Source: CAD feature listing. Evaluate the final solid. Frame: model axes, mm. A direction names the side the tool comes from. Give positions to 0.01 mm unless a question says otherwise; leave off trailing zeros. Loops run counter-clockwise (first coordinate to the right, second up) from the corner with the lowest first, then second, coordinate; pieces in that order, holes last. Notation, with made-up numbers: M 51,-16.75 L 77,-16.75 A9 ccw 77,-4.75 Z; hole C 44,42 d6. An arc over 180 degrees is marked long. Answer in a Markdown table with one row per item.
Autodesk Inventor part; units mm, degrees
ref_plane "YZ Plane" through (0, 0, 0) normal (1, 0, 0) x (0, 1, 0)
ref_plane "XZ Plane" through (0, 0, 0) normal (0, 1, 0) x (-1, 0, 0)
ref_plane "XY Plane" through (0, 0, 0) normal (0, 0, 1) x (1, 0, 0)
sketch "草圖1" plane through (0, 0, 0) normal (0, 1, 0) x (-1, 0, 0)
  line L0 (0, 0) -> (42, 0)
  line L1 (42, 0) -> (42, 12)
  line L2 (42, 12) -> (0, 12)
  line L3 (0, 12) -> (0, 0)
  line L4 (0, 0) -> (-8.5, 0)
  line L5 (-10, 1.5) -> (-10, 1.5)
  line L6 (-8.5, 3) -> (0, 3)
  line L7 (0, 3) -> (0, 0)
  line L8 (30, 0) -> (42, 0)
  line L9 (42, 0) -> (42, -6)
  line L10 (36, -12) -> (36, -12)
  line L11 (30, -6) -> (30, 0)
  arc A0 (30, -6) -> (36, -12) centre (36, -6) ccw
  arc A1 (36, -12) -> (42, -6) centre (36, -6) ccw
  arc A2 (-8.5, 3) -> (-10, 1.5) centre (-8.5, 1.5) ccw
  arc A3 (-10, 1.5) -> (-8.5, 0) centre (-8.5, 1.5) ccw
  point P0 (-10, 3)
  point P1 (-10, 0)
  point P2 (42, -12)
  point P3 (30, -12)
  dimension "d0" = 42
  dimension "d2" = 10
  dimension "d3" = 3
  dimension "d4" = 12
  dimension "d6" = 12
  dimension "d7" = 12
  dimension "d8" = 6
  dimension "d9" = 1.5
extrude "擠出1" add sketch "草圖1" along normal blind 12
fillet "圓角1" radius 3 4 edges at (-42, 6, 12) (-30, 6, 0) (0, 6, 3) (0, 6, 12)
sketch "草圖2" plane through (0, 12, 0) normal (0, 1, 0) x (1, 0, 0)
  line L0 (-42, 6) -> (-42, -9)
  line L1 (-39, -12) -> (-3, -12)
  point P0 (0, 0)
  point P1 (-36, -6)
  dimension "d13" = 6
  dimension "d14" = 6
hole "孔1" at (-36, 12, 6) direction (0, -1, 0) diameter 3 end through all counterbore diameter 7 counterbore depth 2
sketch "草圖3" plane through (8.5, 0, 0) normal (0, 0, -1) x (-1, 0, 0)
  line L0 (35.5, 12) -> (35.5, 0)
  line L1 (0, 0) -> (35.5, 0)
  line L2 (35.5, 9) -> (50.5, 9)
  line L3 (50.5, 9) -> (50.5, 3)
  line L4 (50.5, 3) -> (35.5, 3)
  line L5 (35.5, 3) -> (35.5, 9)
  point P0 (8.5, 0)
  dimension "d22" = 6
  dimension "d24" = 15
  dimension "d25" = 3
extrude "擠出2" cut sketch "草圖3" along normal blind 12
sketch "草圖4" plane through (0, 12, 0) normal (0, 1, 0) x (1, 0, 0)
  line L0 (-30, 3) -> (-30, 6)
  point P0 (0, 0)
  point P1 (-34, 6)
  dimension "d28" = 4
hole "孔2" at (-34, 12, -6) direction (0, -1, 0) diameter 3.242 end through all counterbore diameter 7.5 counterbore depth 2
sketch "草圖5" plane through (-39, 0, 12) normal (0, 0, 1) x (1, 0, 0)
  line L0 (-3, 12) -> (-3, 0)
  point P0 (39, 0)
  point P1 (12, 6)
  dimension "d36" = 15
hole "孔3" at (-27, 6, 12) direction (0, 0, -1) diameter 2.5 end through all
chamfer "倒角1" distance 0.25 angle 45 2 edges at (-27, 7.25, 12) (-27, 7.25, 0)
sketch "草圖6" plane through (-39, 0, 12) normal (0, 0, 1) x (1, 0, 0)
  line L0 (-3, 12) -> (-3, 0)
  point P0 (39, 0)
  point P1 (29, 6)
  dimension "d47" = 32
hole "孔4" at (-10, 6, 12) direction (0, 0, -1) diameter 3.242 end through all
properties part number "extruder_lever"
1) Material intervals for L1, parallel to Z at x = -36, y = 8.5; L2, parallel to Y at x = -27, z = 5.5; L3, parallel to Z at x = -23, y = 2.5, sorted ascending.
Reply:
| item | result |
|---|---|
| L1 | z = 0 to 4.5, 7.5 to 12 |
| L2 | y = 0 to 4.75, 7.25 to 12 |
| L3 | z = 0 to 12 |
2) Section D-D, the plane z = 3.75. Return loops of the section in (x, y).
Reply:
| item | result |
|---|---|
| outline | M -42,0 L 1.02,0 L 1.02,12 L -33.32,12 L -33.32,10 L -38.68,10 L -38.68,12 L -42,12 Z; hole C -27,6 d2.5; hole C -10,6 d3.24 |
3) Section A-A, the plane y = 6. Return loops of the section in (x, z).
Reply:
| item | result |
|---|---|
| outline | M -42,0 L -28.5,0 L -28.25,0.25 L -28.25,11.75 L -28.5,12 L -39,12 A3 ccw -42,9 Z; M -25.75,0.25 L -25.5,0 L -11.62,0 L -11.62,12 L -25.5,12 L -25.75,11.75 Z; M -8.38,0 L 8.5,0 A1.5 ccw 8.5,3 L 3,3 A3 cw 0,6 L 0,9 A3 ccw -3,12 L -8.38,12 Z; hole C -36,6 d3 |
4) Set-up query: faces 1 (the flat face through (-16, 6, 0)), 2 (the cylindrical face through (-39.47, 10.99, 5.54)), 3 (the flat face through (-30, 10, -5)), 4 (the flat face through (6, 6, 3)). Return all of +Z, -Z, +X, -X, +Y, -Y with unobstructed straight access to the full face (end or side cutting, diameter ignored); none if empty.
Reply:
| item | result |
|---|---|
| face 1 | -Z, +X |
| face 2 | +Y |
| face 3 | -Z, +X, +Y, -Y |
| face 4 | +Z, +X, +Y, -Y |
5) Section B-B, the plane x = -10. Return loops of the section in (y, z).
Reply:
| item | result |
|---|---|
| outline | M 0,0 L 4.38,0 L 4.38,12 L 0,12 Z; M 7.62,0 L 12,0 L 12,12 L 7.62,12 Z |
6) Pin query (flat end, axial travel): pin 1 Ø3.5 at (y, z) = (2, -4.5) entering from +X; pin 2 Ø1.5 at (y, z) = (4, 7.5) entering from +X; pin 3 Ø5 at (x, z) = (-34, -6) entering from +Y; pin 4 Ø1.8 at (x, z) = (-36, 6) entering from -Y. Return the tip coordinate at first contact, or that it passes through.
Reply:
| item | result |
|---|---|
| pin 1 | stops at x = -29.99 |
| pin 2 | stops at x = 0 |
| pin 3 | stops at y = 10 |
| pin 4 | passes through |
7) Pull-direction query (Y, two-part tool) for faces 5 (the flat face through (-21, 12, 3)), 6 (the cylindrical face through (-32.418, 9.493, -6.351)), 7 (the flat face through (-36, 9, -6)); classes: released by +Y, released by -Y, zero draft, split by the parting line, or undercut.
Reply:
| item | result |
|---|---|
| face 5 | released by +Y |
| face 6 | zero draft |
| face 7 | undercut |
8) Section C-C, the plane y = 8.5. Return loops of the section in (x, z).
Reply:
| item | result |
|---|---|
| outline | M -42,0 L 8.5,0 A1.5 ccw 8.5,3 L 3,3 A3 cw 0,6 L 0,9 A3 ccw -3,12 L -39,12 A3 ccw -42,9 Z; hole C -36,6 d3 |
